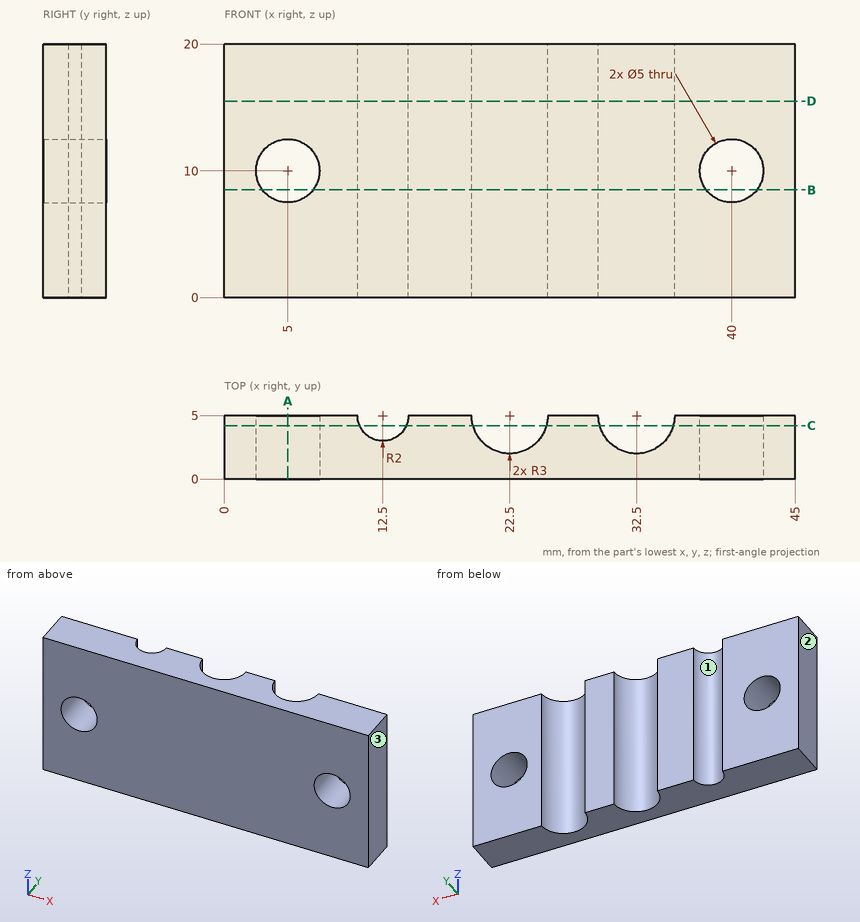
The figure shows three views and two pictorial views of one solid part (mm, origin at its lowest corner). Answer the questions. Round coordinates to 2 decimals unless told otherwise and drop trailing zeros. Write each loop counter-clockwise with the first axis right and the second up, starting at its lowest first coordinate (ties: lowest second). Pieces come first, ordered by that corner, then holes. Notation, with made-up numbers: (10, 42.5) - (44, 42.5) arc R20 cw to (44, 71.5) - close; hole circle Ø4 at (61.25, 18). An arc over 180 degrees is marked (long way). Use one line per item in the form item = value. Start each with the question number.
Item 1: A cutting plane is placed at D-D (z = 15.5). Write down the section's boundary in (x, y), plus the area to 3 significant figures.
Item 2: A cutting plane is placed at C-C (y = 4.2). Write down the section's boundary in (x, z), plus the area to 3 significant figures.
Item 3: Determine the mould class of the marked faces 1, 2 and 3 for opening direction X: +X half, -X half, draft (parallel to the pull), parting line (faces both ways), or undercut.
Item 4: A cutting plane is placed at A-A (x = 5). Write down the section's boundary in (y, z).
Item 5: A cutting plane is placed at B-B (z = 8.5). Write down the section's boundary in (x, y).
Item 6: Find the intervals of material crossed by line 1 (X direction, y = 1.6, z = 10); line 2 (Z direction, x = 40, y = 3.3); line 3 (X direction, y = 3.6, z = 1.25), in increasing order. Write a range as [from, to].
Item 7: Flat-ended cylindrical pins translate along their axes: pin 1 Ø1 at (x, y) = (25.5, 1.5) entering from -Z; pin 2 Ø4 at (x, z) = (40, 10) entering from +Y; pin 3 Ø1.5 at (x, z) = (12.5, 10.5) entering from +Y. Find the tip coordinate at first contact, or state that the pin passes through.
The answers:
q1.outline = (0, 0) - (45, 0) - (45, 5) - (35.5, 5) arc R3 cw to (29.5, 5) - (25.5, 5) arc R3 cw to (19.5, 5) - (14.5, 5) arc R2 cw to (10.5, 5) - (0, 5) - close
q1.area = 190 mm^2
q2.outline = (0, 0) - (10.67, 0) - (10.67, 20) - (0, 20) - close; (14.33, 0) - (19.61, 0) - (19.61, 20) - (14.33, 20) - close; (25.39, 0) - (29.61, 0) - (29.61, 20) - (25.39, 20) - close; (35.39, 0) - (45, 0) - (45, 20) - (35.39, 20) - close; hole circle Ø5 at (5, 10); hole circle Ø5 at (40, 10)
q2.area = 556 mm^2
q3.face_1 = undercut
q3.face_2 = -X half
q3.face_3 = +X half
q4.outline = (0, 0) - (5, 0) - (5, 7.5) - (0, 7.5) - close; (0, 12.5) - (5, 12.5) - (5, 20) - (0, 20) - close
q5.outline = (0, 0) - (3, 0) - (3, 5) - (0, 5) - close; (7, 0) - (38, 0) - (38, 5) - (35.5, 5) arc R3 cw to (29.5, 5) - (25.5, 5) arc R3 cw to (19.5, 5) - (14.5, 5) arc R2 cw to (10.5, 5) - (7, 5) - close; (42, 0) - (45, 0) - (45, 5) - (42, 5) - close
q6.line_1 = [0, 2.5], [7.5, 37.5], [42.5, 45]
q6.line_2 = [0, 7.5], [12.5, 20]
q6.line_3 = [0, 11.07], [13.93, 19.85], [25.15, 29.85], [35.15, 45]
q7.pin_1 = 0
q7.pin_2 = through
q7.pin_3 = 3.15
